```python
from build123d import *

# Parameters (mm, degrees)
F1_DEPTH = 40
F0_W     = 25
F0_H     = 15
F2_DEPTH = 25


with BuildPart() as f1:
    # F0 (on Right) → F1 (new body, symmetric)
    with BuildSketch(Plane.YZ):
        Polygon((-50, -15), (50, -15), (50, 15), (35, 15), (-50, 15), align=None)
    extrude(amount=F1_DEPTH, both=True)

    # F0 (on Right) → F2 (join, symmetric)
    with BuildSketch(Plane.YZ):
        with BuildLine():
            add(Edge.make_bspline(
                [(-50, 15), (-50.800499, 51.844761), (17.916949, 72.011843), (69.400141, 72.759509)],
                knots=[0, 0, 0, 0, 132.636927, 132.636927, 132.636927, 132.636927], degree=3))
            Line((-50, 15), (35, 15))
            Line((35, 15), (35, 37.76465))
            ThreePointArc((35, 37.76465), (45.040081, 62.300388), (69.400141, 72.759509))
        make_face()
        with BuildLine():
            Line((35, 15), (50, 15))
            Line((50, 15), (50, 37.76465))
            ThreePointArc((50, 37.76465), (55.698448, 51.745552), (69.546562, 57.759509))
            Line((69.546562, 57.759509), (75, 57.759509))
            Line((75, 57.759509), (75, 72.759509))
            Line((75, 72.759509), (69.400141, 72.759509))
            ThreePointArc((69.400141, 72.759509), (45.040081, 62.300388), (35, 37.76465))
            Line((35, 37.76465), (35, 15))
        make_face()
        with Locations((87.5, 65.259509)):
            Rectangle(F0_W, F0_H)
    extrude(amount=F2_DEPTH, both=True)

    # F0 (on Right) → F3 (revolve)
    with BuildSketch(Plane.YZ):
        Polygon((100, 77.759509), (100, 72.759509), (100, 57.759509), (100, 52.759509), (125, 52.759509), (125, 77.759509), align=None)
    revolve(axis=Axis((0, 100, 65.259509), (0, 0, -1)))


solid = f1.part
```
Read the model definition and answer for the solid it produces. Units are mm, in the model's axes. A direction names the side the tool comes from. Give positions to 0.01 mm unless a question says otherwise; leave off trailing zeros. Loops run counter-clockwise (first coordinate to the right, second up) from the corner with the lowest first, then second, coordinate; pieces in that order, holes last.
Item 1: The mould has two halves that part along Y. Classify faces 6 (the flat face through (1, 50, 5)), 7 (the flat face through (-32, 1, 15)), 8 (the flat face through (-1.7, 74.6, 57.76)): released by +Y, released by -Y, zero draft, split by the parting line, or undercut.
Item 2: Find the intervals of material crossed by line 1 along Z through (x, y) = (-30, -15.5); line 2 along Y through (x, z) = (-7, 7); line 3 along X through (y, z) = (8, 33.5), in increasing order.
Item 3: For faces 1 (the flat face through (-25, 26, 44)), 2 (the flat face through (0, 100, 52.76)), 3 (the cylindrical face through (0.35, 55.55, 51.59)), 4 (the flat face through (33, 1, 15)), 5 (the cylindrical face through (-9.58, 123.09, 65.43)), determine the directions among +Z, -Z, +X, -X, +Y, -Y from which every point of the face is accessible in a straight line to the end or side of a thin tool.
Item 4: Each of these flat-tipped pins is pushed along its axis until it touches: pin 1 Ø12 at (x, z) = (-4.5, 51.5) entering from -Y; pin 2 Ø1 at (x, z) = (-9.5, 18) entering from +Y; pin 3 Ø1 at (x, y) = (8, 56) entering from +Z. Where does it stop, or does it pass through?
Item 5: The part is cut by section A-A (x = -32). Write down the section's boundary in (y, z).
Item 6: The part is cut by section B-B (z = 8). Write down the section's boundary in (x, y), and give its area (3 significant figures).
Taken from the geometry:
1. face 6: released by +Y
1. face 7: zero draft
1. face 8: undercut
2. line 1: z = -15 to 15
2. line 2: y = -50 to 50
2. line 3: x = -25 to 25
3. face 1: +Z, -X, +Y, -Y
3. face 2: -Z, +X, -X, +Y
3. face 3: -Z, +X, -X
3. face 4: +Z, +X, +Y, -Y
3. face 5: none
4. pin 1: stops at y = -31.79
4. pin 2: stops at y = 50
4. pin 3: stops at z = 72.19
5. outline: (-50, -15) - (50, -15) - (50, 15) - (-50, 15) - close
6. outline: (-40, -50) - (40, -50) - (40, 50) - (-40, 50) - close
6. area: 8,000 mm2
